Input: part model. Units: mm. Frame: model coordinates. A direction names the side the tool comes from. Round coordinates to 2 decimals unless told otherwise and drop trailing zeros. Write each loop counter-clockwise with the first axis right and the second up, starting at its lowest first coordinate (ties: lowest second). Pieces come first, ordered by that corner, then holes. Notation, with made-up numbers: (64, 10.5) -> (114, 10.5) arc R11 ccw to (114, 16.5) -> close; hole circle Ø8 at (-23.5, -31.75). An arc over 180 degrees is marked (long way). Use CSV: the item, a comma, the result in double quotes.
```python
from build123d import *

# Parameters (mm, degrees)
CROQUIS11_W             = 27.4
CROQUIS11_H             = 49.26
SALIENTE_EXTRUIR3_DEPTH = 3
CORTAR_EXTRUIR1_DEPTH   = 56
SALIENTE_EXTRUIR4_DEPTH = 49.26
CROQUIS24_W             = 25.4
CROQUIS24_H             = 1
SALIENTE_EXTRUIR6_DEPTH = 2
SALIENTE_EXTRUIR7_DEPTH = 2


with BuildPart() as part:
    # Croquis11 → Saliente-Extruir3 (new body)
    with BuildSketch(Plane(origin=(0, 0, 0), x_dir=(1, 0, 0), z_dir=(0, 1, 0))):
        Rectangle(CROQUIS11_W, CROQUIS11_H)
    extrude(amount=SALIENTE_EXTRUIR3_DEPTH)

    # Croquis21 → Cortar-Extruir1 (cut)
    with BuildSketch(Plane(origin=(0, 0, -24.63), x_dir=(-1, 0, 0), z_dir=(0, 0, -1))):
        Polygon((-12.7, 2), (-13.7, 2), (-13.7, 1.5), (-13.7, 1), (-12.7, 1), (-12.7, 1.5), align=None)
        Polygon((13.7, 2), (12.7, 2), (12.7, 1.5), (12.7, 1), (13.7, 1), (13.7, 1.5), align=None)
    extrude(amount=-CORTAR_EXTRUIR1_DEPTH, mode=Mode.SUBTRACT)

    # Croquis23 → Saliente-Extruir4 (add)
    with BuildSketch(Plane.XY.offset(24.63)):
        Polygon((-13.7, 5), (-13.7, 3), (-12.7, 3), (-12.7, 4), (-11.7, 4), (-11.7, 5), align=None)
        Polygon((12.7, 4), (12.7, 3), (13.7, 3), (13.7, 5), (11.7, 5), (11.7, 4), align=None)
    extrude(amount=-SALIENTE_EXTRUIR4_DEPTH)

    # Croquis24 → Saliente-Extruir6 (add)
    with BuildSketch(Plane(origin=(0, 3, 0), x_dir=(1, 0, 0), z_dir=(0, 1, 0))):
        with Locations((0, -24.13)):
            Rectangle(CROQUIS24_W, CROQUIS24_H)
    extrude(amount=SALIENTE_EXTRUIR6_DEPTH)

    # Croquis26 → Saliente-Extruir7 (add)
    with BuildSketch(Plane(origin=(0, 5, 0), x_dir=(1, 0, 0), z_dir=(0, 1, 0))):
        Polygon((-13.7, 24.63), (-11.7, 24.63), (-11.7, -23.63), (11.7, -23.63), (11.7, 24.63), (13.7, 24.63), (13.7, -24.63), (-13.7, -24.63), align=None)
    extrude(amount=SALIENTE_EXTRUIR7_DEPTH)


solid = part.part
```
Item 1: Set-up query: faces 5 (the face through (12.7, 3.5, -0.2)), 6 (the face through (-13.7, 0.5, 0.3)), 7 (the face through (-13, 2, 0)), 8 (the face through (12, 7, 0)), 9 (the face through (11.7, 6, 0)). Return all of +Z, -Z, +X, -X, +Y, -Y with unobstructed straight access to the full face (end or side cutting, diameter ignored); none if empty.
Worked answers:
face 5,"-Z"
face 6,"+Z, -Z, -X, +Y, -Y"
face 7,"+Z, -Z, -X"
face 8,"+Z, -Z, +X, -X, +Y"
face 9,"-Z, +Y"
Item 2: Section query A-A on y = 5.75. Return the cut outline in (x, z), plus the area to 3 significant figures.
Worked answers:
outline,"(-13.7, -24.63) -> (-11.7, -24.63) -> (-11.7, 23.63) -> (11.7, 23.63) -> (11.7, -24.63) -> (13.7, -24.63) -> (13.7, 24.63) -> (-13.7, 24.63) -> close"
area,"220 mm²"
Item 3: Section query B-B on x = 5.75. Return the cut outline in (y, z).
Worked answers:
outline,"(0, -24.63) -> (3, -24.63) -> (3, 23.63) -> (7, 23.63) -> (7, 24.63) -> (0, 24.63) -> close"
Item 4: First-contact query: pin 1 Ø2 at (x, y) = (-3.5, 5) entering from -Z; pin 2 Ø0.8 at (y, z) = (1.5, -11) entering from -X. Flat tips, straight axial feed; report the tip coordinate or a pass-through.
Worked answers:
pin 1,"stops at z = 23.63"
pin 2,"stops at x = -12.7"
Item 5: Section query D-D on y = 1.5. Return the cut outline in (x, z), plus the area to 3 significant figures.
Worked answers:
outline,"(-12.7, -24.63) -> (12.7, -24.63) -> (12.7, 24.63) -> (-12.7, 24.63) -> close"
area,"1,250 mm²"
Item 6: Pull-direction query (Y, two-part tool) for faces 1 (the face through (0, 0, 0)), 2 (the face through (12.7, 1.5, -0.3)), 3 (the face through (13.7, 4, 0)), 4 (the face through (13, 1, 0)); classes: +Y half, -Y half, draft (parallel to the pull), parting line (faces both ways), or undercut.
Worked answers:
face 1,"-Y half"
face 2,"undercut"
face 3,"draft"
face 4,"undercut"
Item 7: Line query: line 1 (X direction, y = 5.5, z = 9); line 2 (Z direction, x = -2.75, y = 4); line 3 (Y direction, x = -8, z = -1.5). Output: solid intervals per line, ascending.
Worked answers:
line 1,"x = -13.7 to -11.7, 11.7 to 13.7"
line 2,"z = 23.63 to 24.63"
line 3,"y = 0 to 3"
Item 8: Section query C-C on z = -14. Return the cut outline in (x, y).
Worked answers:
outline,"(-13.7, 0) -> (13.7, 0) -> (13.7, 1) -> (12.7, 1) -> (12.7, 2) -> (13.7, 2) -> (13.7, 7) -> (11.7, 7) -> (11.7, 4) -> (12.7, 4) -> (12.7, 3) -> (-12.7, 3) -> (-12.7, 4) -> (-11.7, 4) -> (-11.7, 7) -> (-13.7, 7) -> (-13.7, 2) -> (-12.7, 2) -> (-12.7, 1) -> (-13.7, 1) -> close"
